```python
from build123d import *

# Parameters (mm, degrees)
BOSS_EXTRUDE1_DEPTH = 15
SKETCH2_R           = 2
CUT_EXTRUDE1_DEPTH  = 34.778691508
SKETCH3_W           = 25.9
SKETCH3_H           = 8
BOSS_EXTRUDE2_DEPTH = 20


with BuildPart() as part:
    # Sketch1 → Boss-Extrude1 (new body)
    with BuildSketch(Plane(origin=(0, 0, 0), x_dir=(1, 0, 0), z_dir=(0, 1, 0))):
        with BuildLine():
            Line((-30, -4), (0, -4))
            ThreePointArc((0, -4), (-4, 0), (0, 4))
            Line((0, 4), (-30, 4))
            Line((-30, 4), (-30, -4))
        make_face()
        with BuildLine():
            ThreePointArc((0, 4), (-4, 0), (0, -4))
            Line((0, -4), (0, 4))
        make_face()
        with BuildLine():
            Line((0, 4), (0, -4))
            ThreePointArc((0, -4), (2.828427125, -2.828427125), (4, 0))
            ThreePointArc((4, 0), (2.828427125, 2.828427125), (0, 4))
        make_face()
    extrude(amount=BOSS_EXTRUDE1_DEPTH)

    # Sketch2 → Cut-Extrude1 (cut, through all)
    with BuildSketch(Plane(origin=(0, 15, 0), x_dir=(1, 0, 0), z_dir=(0, 1, 0))):
        with Locations(Location((0, 0, 0), (0, 0, 270))):
            Circle(SKETCH2_R)
    extrude(amount=-CUT_EXTRUDE1_DEPTH, mode=Mode.SUBTRACT)

    # Sketch3 → Boss-Extrude2 (add)
    with BuildSketch(Plane.XZ):
        with Locations((-17.05, 0)):
            Rectangle(SKETCH3_W, SKETCH3_H)
    extrude(amount=BOSS_EXTRUDE2_DEPTH)


solid = part.part
```
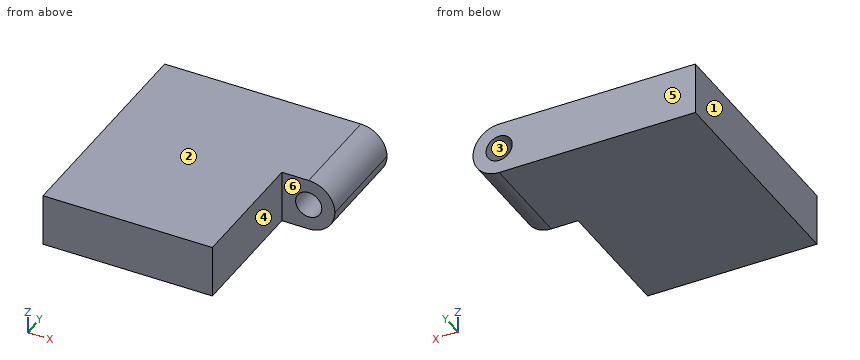
The model under review builds one solid part; all positions refer to its coordinate system, in mm. Face numbers are marked on the shaded views. A direction names the side the tool comes from. Round coordinates to 2 decimals unless told otherwise and drop trailing zeros. Order: outer loops, then holes, each group sorted by start corner. A loop starts at its lowest first (then second) coordinate and runs counter-clockwise, first axis right, second up. Notation, with made-up numbers: (81, -1.75) -> (88, -1.75) arc R18 cw to (88, 21.25) -> close; hole circle Ø2 at (-4, 54). An arc over 180 degrees is marked (long way). One line per item, written item: value. Start each with the question number.
Q1. Clearance check with flat-ended pins moving along their axes: pin 1 Ø1 at (y, z) = (-1, -0.5) entering from +X; pin 2 Ø4 at (x, z) = (-0.5, 1.5) entering from -Y; pin 3 Ø1.5 at (y, z) = (8.5, -2) entering from +X. State where each tip first meets the part, or that it passes through.
Q2. Take a section at B-B (z = 2.75). Write out the cut boundary in (x, y).
Q3. Machinability: for the marked faces 5 and 6, which of the approach directions +Z, -Z, +X, -X, +Y, -Y give a long, thin tool a straight path to every point of the face, cutting with its end or side? Answer none if there is none.
Q4. Mouldability with a two-part tool opening along X and no side actions: class the marked faces 1, 2, 3 and 4 as released by +X, released by -X, zero draft, split by the parting line, or undercut.
Q5. Take a section at A-A (y = 1.5). Write out the cut boundary in (x, z).
Q6. Take a section at C-C (y = -14). Write out the cut boundary in (x, z).
Q7. Wall thickness on line 1 (Y direction, x = 2.5, z = 0.25); line 2 (X direction, y = -17.5, z = 0); line 3 (X direction, y = 12, z = -1.75): over which ranges is each line inside the solid? List them lowest first.
Reported:
1. pin 1: stops at x = -4.1
1. pin 2: stops at y = 0
1. pin 3: stops at x = 3.8
2. outline: (-30, -20) -> (-4.1, -20) -> (-4.1, 0) -> (2.9, 0) -> (2.9, 15) -> (-30, 15) -> close
3. face 5: +Z, -Z, +X, -X, +Y
3. face 6: +Z, -Z, +X, -Y
4. face 1: released by -X
4. face 2: zero draft
4. face 3: undercut
4. face 4: released by +X
5. outline: (-30, -4) -> (0, -4) arc R4 ccw to (0, 4) -> (-30, 4) -> close; hole circle Ø4 at (0, 0)
6. outline: (-30, -4) -> (-4.1, -4) -> (-4.1, 4) -> (-30, 4) -> close
7. line 1: y = 0 to 15
7. line 2: x = -30 to -4.1
7. line 3: x = -30 to -0.97, 0.97 to 3.6
